Read the model definition and answer for the solid it produces. Units are mm, in the model's axes. A direction names the side the tool comes from. Give positions to 0.01 mm unless a question says otherwise; leave off trailing zeros. Write each loop counter-clockwise with the first axis right and the second up, starting at its lowest first coordinate (ties: lowest second). Pieces come first, ordered by that corner, then holes. Notation, with made-up numbers: M 63,7.25 L 99,7.25 A25 ccw 99,31.25 Z; hole C -18,3 d1. An arc over 180 degrees is marked long. Put each result on its own line as item: value.
from build123d import *

# Parameters (mm, degrees)
SKETCH1_R               = 43.5
SKETCH1_R_2             = 40.5
BOSS_EXTRUDE1_DEPTH     = 30
SKETCH2_R               = 43.5
SKETCH2_R_2             = 40.5
BOSS_EXTRUDE2_DEPTH     = 20
BOSS_EXTRUDE3_START     = 5
SKETCH3_R               = 43.5
SKETCH3_R_2             = 40.5
BOSS_EXTRUDE3_DEPTH     = 5
CUT_EXTRUDE1_DEPTH      = 10
CUT_EXTRUDE1_DEPTH_BACK = 10


with BuildPart() as part:
    # Sketch1 → Boss-Extrude1 (new body)
    # profile 1 of 5: a face of its own
    with BuildSketch(Plane(origin=(0, 0, 0), x_dir=(1, 0, 0), z_dir=(0, 1, 0))):
        with Locations(Location((0, 0, 0), (0, 0, 270))):
            Circle(SKETCH1_R)
        Circle(SKETCH1_R_2, mode=Mode.SUBTRACT)
    # profile 2 of 5: a face of its own
    with BuildSketch(Plane(origin=(0, 0, 0), x_dir=(1, 0, 0), z_dir=(0, 1, 0))):
        with BuildLine():
            ThreePointArc((-29.123002918, 28.14428363), (-20.35009445, 28.49013223), (-17.177672758, 36.676662316))
            ThreePointArc((-17.177672758, 36.676662316), (-23.540146846, 32.956205584), (-29.123002918, 28.14428363))
        make_face()
    # profile 3 of 5: a face of its own
    with BuildSketch(Plane(origin=(0, 0, 0), x_dir=(1, 0, 0), z_dir=(0, 1, 0))):
        with BuildLine():
            ThreePointArc((-29.123002918, -28.14428363), (-23.540146846, -32.956205584), (-17.177672758, -36.676662316))
            ThreePointArc((-17.177672758, -36.676662316), (-20.35009445, -28.49013223), (-29.123002918, -28.14428363))
        make_face()
    # profile 4 of 5: a face of its own
    with BuildSketch(Plane(origin=(0, 0, 0), x_dir=(1, 0, 0), z_dir=(0, 1, 0))):
        with BuildLine():
            ThreePointArc((17.177672758, -36.676662316), (23.540146846, -32.956205584), (29.123002918, -28.14428363))
            ThreePointArc((29.123002918, -28.14428363), (20.35009445, -28.49013223), (17.177672758, -36.676662316))
        make_face()
    # profile 5 of 5: a face of its own
    with BuildSketch(Plane(origin=(0, 0, 0), x_dir=(1, 0, 0), z_dir=(0, 1, 0))):
        with BuildLine():
            ThreePointArc((17.177672758, 36.676662316), (20.35009445, 28.49013223), (29.123002918, 28.14428363))
            ThreePointArc((29.123002918, 28.14428363), (23.540146846, 32.956205584), (17.177672758, 36.676662316))
        make_face()
    extrude(amount=BOSS_EXTRUDE1_DEPTH)

    # Sketch2 → Boss-Extrude2 (add)
    with BuildSketch(Plane(origin=(0, 30, 0), x_dir=(1, 0, 0), z_dir=(0, 1, 0))):
        with Locations(Location((0, 0, 0), (0, 0, 270))):
            Circle(SKETCH2_R)
        with Locations(Location((0, 0, 0), (0, 0, 64.90375534))):
            Circle(SKETCH2_R_2, mode=Mode.SUBTRACT)
    extrude(amount=BOSS_EXTRUDE2_DEPTH)

    # Sketch3 → Boss-Extrude3 (add)
    with BuildSketch(Plane.XZ.offset(BOSS_EXTRUDE3_START)):
        with Locations(Location((0, 0, 0), (0, 0, 270))):
            Circle(SKETCH3_R)
        with Locations(Location((0, 0, 0), (0, 0, 270))):
            Circle(SKETCH3_R_2, mode=Mode.SUBTRACT)
    extrude(amount=-BOSS_EXTRUDE3_DEPTH)

    # Sketch5 → Cut-Extrude1 (cut, two sides: drawn at the far end of the back side and taken through both)
    with BuildSketch(Plane(origin=(0, 15, 0), x_dir=(1, 0, 0), z_dir=(0, 1, 0)).offset(-CUT_EXTRUDE1_DEPTH_BACK)):
        with BuildLine():
            ThreePointArc((-4.991735805, 43.212643678), (-4.654531608, 41.673709906), (-3.855221077, 40.316091954))
            ThreePointArc((-3.855221077, 40.316091954), (0, 40.5), (3.855221077, 40.316091954))
            ThreePointArc((3.855221077, 40.316091954), (4.654531608, 41.673709906), (4.991735805, 43.212643678))
            ThreePointArc((4.991735805, 43.212643678), (0, 43.5), (-4.991735805, 43.212643678))
        make_face()
        with BuildLine():
            ThreePointArc((33.924080965, 22.122538974), (31.66417504, 25.251336975), (29.116698914, 28.150805394))
            ThreePointArc((29.116698914, 28.150805394), (29.679765405, 29.622192479), (30.6727089, 30.845338849))
            ThreePointArc((30.6727089, 30.845338849), (34.009669487, 27.121806381), (36.897301636, 23.03994644))
            ThreePointArc((36.897301636, 23.03994644), (35.483871385, 22.344073784), (33.924080965, 22.122538974))
        make_face()
        with BuildLine():
            ThreePointArc((40.163150751, 5.212611799), (39.484580443, 9.012097825), (38.447415961, 12.729737071))
            ThreePointArc((38.447415961, 12.729737071), (39.59313227, 13.811105632), (41.018446768, 14.482300396))
            ThreePointArc((41.018446768, 14.482300396), (42.40936418, 9.679660627), (43.239978194, 4.749135264))
            ThreePointArc((43.239978194, 4.749135264), (41.664593712, 4.735440067), (40.163150751, 5.212611799))
        make_face()
        with BuildLine():
            ThreePointArc((41.018446768, -14.482300396), (42.40936418, -9.679660627), (43.239978194, -4.749135264))
            ThreePointArc((43.239978194, -4.749135264), (41.664593712, -4.735440067), (40.163150751, -5.212611799))
            ThreePointArc((40.163150751, -5.212611799), (39.484580443, -9.012097825), (38.447415961, -12.729737071))
            ThreePointArc((38.447415961, -12.729737071), (39.59313227, -13.811105632), (41.018446768, -14.482300396))
        make_face()
        with BuildLine():
            ThreePointArc((29.116698914, -28.150805394), (29.679765405, -29.622192479), (30.6727089, -30.845338849))
            ThreePointArc((30.6727089, -30.845338849), (34.009669487, -27.121806381), (36.897301636, -23.03994644))
            ThreePointArc((36.897301636, -23.03994644), (35.483871385, -22.344073784), (33.924080965, -22.122538974))
            ThreePointArc((33.924080965, -22.122538974), (31.66417504, -25.251336975), (29.116698914, -28.150805394))
        make_face()
        with BuildLine():
            ThreePointArc((4.991735805, -43.212643678), (4.654531608, -41.673709906), (3.855221077, -40.316091954))
            ThreePointArc((3.855221077, -40.316091954), (0, -40.5), (-3.855221077, -40.316091954))
            ThreePointArc((-3.855221077, -40.316091954), (-4.654531608, -41.673709906), (-4.991735805, -43.212643678))
            ThreePointArc((-4.991735805, -43.212643678), (0, -43.5), (4.991735805, -43.212643678))
        make_face()
        with BuildLine():
            ThreePointArc((-36.897301636, -23.03994644), (-34.009669487, -27.121806381), (-30.6727089, -30.845338849))
            ThreePointArc((-30.6727089, -30.845338849), (-29.679765405, -29.622192479), (-29.116698914, -28.150805394))
            ThreePointArc((-29.116698914, -28.150805394), (-31.66417504, -25.251336975), (-33.924080965, -22.122538974))
            ThreePointArc((-33.924080965, -22.122538974), (-35.483871385, -22.344073784), (-36.897301636, -23.03994644))
        make_face()
        with BuildLine():
            ThreePointArc((-43.239978194, -4.749135264), (-42.40936418, -9.679660627), (-41.018446768, -14.482300396))
            ThreePointArc((-41.018446768, -14.482300396), (-39.59313227, -13.811105632), (-38.447415961, -12.729737071))
            ThreePointArc((-38.447415961, -12.729737071), (-39.484580443, -9.012097825), (-40.163150751, -5.212611799))
            ThreePointArc((-40.163150751, -5.212611799), (-41.664593712, -4.735440067), (-43.239978194, -4.749135264))
        make_face()
        with BuildLine():
            ThreePointArc((-38.447415961, 12.729737071), (-39.484580443, 9.012097825), (-40.163150751, 5.212611799))
            ThreePointArc((-40.163150751, 5.212611799), (-41.664593712, 4.735440067), (-43.239978194, 4.749135264))
            ThreePointArc((-43.239978194, 4.749135264), (-42.40936418, 9.679660627), (-41.018446768, 14.482300396))
            ThreePointArc((-41.018446768, 14.482300396), (-39.59313227, 13.811105632), (-38.447415961, 12.729737071))
        make_face()
        with BuildLine():
            ThreePointArc((-29.116698914, 28.150805394), (-29.679765405, 29.622192479), (-30.6727089, 30.845338849))
            ThreePointArc((-30.6727089, 30.845338849), (-34.009669487, 27.121806381), (-36.897301636, 23.03994644))
            ThreePointArc((-36.897301636, 23.03994644), (-35.483871385, 22.344073784), (-33.924080965, 22.122538974))
            ThreePointArc((-33.924080965, 22.122538974), (-31.66417504, 25.251336975), (-29.116698914, 28.150805394))
        make_face()
    extrude(amount=CUT_EXTRUDE1_DEPTH + CUT_EXTRUDE1_DEPTH_BACK, mode=Mode.SUBTRACT)


solid = part.part
(1) Straight lines are drawn through the part: line 1 along Z through (x, y) = (0, 38.5); line 2 along X through (y, z) = (3, 15). For each, find the intervals that lie inside material, in ascending order. Write a range as from..to.
Result:
line 1: z = -43.5..-40.5, 40.5..43.5
line 2: x = -40.83..-37.62, 37.62..40.83
(2) Section C-C on y = 2 is taken. Determine the outline of the cut face in (x, z).
Result:
outline: C 0,0 d87; hole M -29.12,-28.14 A8 cw -17.18,-36.68 A40.5 ccw 17.18,-36.68 A8 cw 29.12,-28.14 A40.5 ccw 29.12,28.14 A8 cw 17.18,36.68 A40.5 ccw -17.18,36.68 A8 cw -29.12,28.14 A40.5 ccw Z
(3) Section B-B on x = 0 is taken. Determine the outline of the cut face in (y, z), and give its area (3 significant figures).
Result:
outline: M -5,-43.5 L 5,-43.5 L 5,-40.5 L -5,-40.5 Z; M -5,40.5 L 5,40.5 L 5,43.5 L -5,43.5 Z; M 25,-43.5 L 50,-43.5 L 50,-40.5 L 25,-40.5 Z; M 25,40.5 L 50,40.5 L 50,43.5 L 25,43.5 Z
area: 210 mm²
(4) Given pin 1 Ø4 at (y, z) = (40.5, 4) entering from +X; pin 2 Ø2 at (y, z) = (31.5, -21.5) entering from -X; pin 3 Ø12 at (x, y) = (-11.5, 39.5) entering from -Z; pin 4 Ø12 at (x, z) = (33.5, 7.5) entering from -Y, each flat-ended and moving along its own axis, determine where each tip first touches the part or whether it passes through.
Result:
pin 1: stops at x = 43.45
pin 2: stops at x = -38.37
pin 3: stops at z = -43.15
pin 4: passes through
(5) For a pull along Z with two mould halves and no side action, classify faces 4 (the face through (41.69, 14.86, -4.73)), 5 (the face through (0, 5, -42)) as +Z half, -Z half, draft (parallel to the pull), parting line (faces both ways), or undercut.
Result:
face 4: undercut
face 5: draft
(6) Section D-D on x = -10.5 is taken. Determine the outline of the cut face in (y, z).
Result:
outline: M -5,-42.21 L 50,-42.21 L 50,-39.12 L -5,-39.12 Z; M -5,39.12 L 50,39.12 L 50,42.21 L -5,42.21 Z
(7) Which of the six approach directions +Z, -Z, +X, -X, +Y, -Y give full straight-line access (tool end or side, diameter ignored) to faces 1 (the face through (-39.611, 14.86, 13.824)), 2 (the face through (39.575, 14.86, -13.799)), 3 (the face through (41.69, 14.86, 4.73))?
Result:
face 1: -X
face 2: +X
face 3: none
(8) Section A-A on z = 0 is taken. Determine the outline of the cut face in (x, y).
Result:
outline: M -43.5,-5 L -40.5,-5 L -40.5,50 L -43.5,50 Z; M 40.5,-5 L 43.5,-5 L 43.5,50 L 40.5,50 Z
